Input: part model. Units: mm. Frame: model coordinates. Coordinates: 2 decimals unless noted, no trailing zeros. Write each loop counter-clockwise with the first axis right and the second up, starting at its lowest first coordinate (ties: lowest second). Pieces come first, ordered by that corner, then holes. Notation, with made-up numbers: M -30.5,-32 L -24.5,-32 A33 ccw -24.5,-4 Z; hole C 36,73.25 d2. An arc over 180 degrees is marked long. Write each question's results on one line, items separated by ' | '. Start each with the question number.
1. First-contact query: pin 1 (3.5 mm diameter, centred on y = -1.5, z = -22.5, fed in from +X); pin 2 (5 mm diameter, centred on x = 331.5, z = 23.5, fed in from -Y); pin 3 (6 mm diameter, centred on x = 244, y = -1.5, fed in from +Z); pin 4 (3.5 mm diameter, centred on x = 151, y = 2, fed in from -Z). Flat tips, straight axial feed; report the tip coordinate or a pass-through.
2. Ray query, probe 1 along Z at (x, y) = (100, 0.5); probe 2 along X at (y, z) = (1.75, -13); probe 3 along X at (y, z) = (-3.75, -15). Return the intervals inside material, ascending.
3. Section query B-B, the plane x = 37.5. Output: boundary loops of the cut face in (y, z), and give its area (3 significant figures).
4. Section query A-A, the plane z = 21.5. Output: boundary loops of the cut face in (x, y).
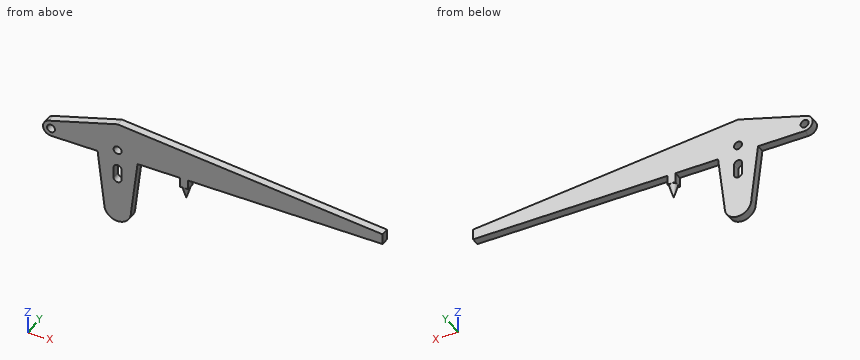
Solid Edge part; units mm, degrees
sketch "Sketch1" plane through (0, 0, 0) normal (0, -1, 0) x (1, 0, 0)
  line L0 (70, -12) -> (0, -12)
  arc A0 (0, -12) -> (-3.4277, 11.5) centre (0, 0) cw
  line L1 (-3.4277, 11.5) -> (100, 42.328)
  line L2 (100, 42.328) -> (498, 4)
  line L3 (498, 4) -> (498, -12)
  line L4 (498, -12) -> (206, -12)
  line L5 (206, -12) -> (206, -26.3599)
  line L6 (206, -26.3599) -> (194, -26.3599)
  line L7 (194, -26.3599) -> (194, -12)
  line L8 (194, -12) -> (130, -12)
  line L9 (130, -12) -> (120, -96.0459)
  arc A1 (120, -96.0459) -> (80, -96.0459) centre (100, -96.0459) cw
  line L10 (80, -96.0459) -> (70, -12)
  circle A2 centre (0, 0) radius 6
  circle A3 centre (100, 0) radius 6
  line L11 (94, -46.3037) -> (94, -30.3037)
  arc A4 (106, -46.3037) -> (94, -46.3037) centre (100, -46.3037) cw
  line L12 (106, -30.3037) -> (106, -46.3037)
  arc A5 (94, -30.3037) -> (106, -30.3037) centre (100, -30.3037) cw
  dimension "D1" = 206
  dimension "D2" = 12
  dimension "D3" = 498
extrude "Protrusion1" add sketch "Sketch1" along normal mid plane 12
sketch "Sketch2" plane through (0, 0, 0) normal (0, -1, 0) x (1, 0, 0)
  line L0 (200, -46) -> (206, -26.3599)
  line L1 (206, -26.3599) -> (200, -26.3599)
revolve "RevolvedProtrusion1" add sketch "Sketch2" angle 360 about axis through (200, 0, -26.3599) along (0, 0, -1)
properties part number "11" material "Fe 410 W"
Answer:
1) pin 1: x = 206 | pin 2: through | pin 3: z = 28.75 | pin 4: z = -12
2) probe 1: -116.05 to -52.3, -24.3 to -6, 6 to 42.33 | probe 2: 70.12 to 129.88, 194 to 206 | probe 3: 70.36 to 129.64, 194 to 206
3) outline: M -6,-12 L 6,-12 L 6,23.7 L -6,23.7 Z | area: 428 mm^2
4) outline: M 30.12,-6 L 316.28,-6 L 316.28,6 L 30.12,6 Z
